from build123d import *

# Parameters (mm, degrees)
PAD006_DEPTH         = 1
SKETCH010_W          = 9.75
SKETCH010_H          = 7
PAD007_DEPTH         = 1.85
SKETCH012_R          = 1.875
PAD005_DEPTH         = 2
POCKET_DEPTH         = 9.001
POCKET001_DEPTH      = 4.876
POCKET001_DEPTH_BACK = -4.876
CHAMFER_SIZE         = 0.3


with BuildPart() as part:
    # Sketch013 → Pad006 (new body)
    with BuildSketch(Plane.XZ):
        with BuildLine():
            ThreePointArc((1.274755, -5.005), (0, -4.505), (-1.274755, -5.005))
            Line((-1.274755, -5.005), (-3.875, -5.005))
            ThreePointArc((-3.875, -5.005), (-4.582107, -5.297893), (-4.875, -6.005))
            Line((-4.875, -6.005), (-4.875, -7.255))
            ThreePointArc((-4.875, -7.255), (-4.582107, -7.962107), (-3.875, -8.255))
            Line((-3.875, -8.255), (3.875, -8.255))
            ThreePointArc((3.875, -8.255), (4.582107, -7.962107), (4.875, -7.255))
            Line((4.875, -7.255), (4.875, -6.005))
            ThreePointArc((4.875, -6.005), (4.582107, -5.297893), (3.875, -5.005))
            Line((3.875, -5.005), (1.274755, -5.005))
        make_face()
    extrude(amount=PAD006_DEPTH)

    # Sketch010 → Pad007 (join)
    with BuildSketch(Plane.XZ):
        with Locations((0, -5.5)):
            Rectangle(SKETCH010_W, SKETCH010_H)
    extrude(amount=-PAD007_DEPTH)

    # Sketch012 → Pad005 (join)
    with BuildSketch(Plane.XZ.offset(1)):
        with Locations((0, -6.38)):
            Circle(SKETCH012_R)
    extrude(amount=PAD005_DEPTH)

    # Sketch → Pocket (cut, through all)
    with BuildSketch(Plane.XY):
        Polygon((-1.275, 3.6), (-1.275, 1.6), (1.275, 1.6), (1.275, 3.6), (4.875, 0), (4.875, 5), (-4.875, 5), (-4.875, 0), align=None)
    extrude(amount=-POCKET_DEPTH, mode=Mode.SUBTRACT)

    # Sketch014 → Pocket001 (cut, two sides)
    with BuildSketch(Plane.YZ) as pocket001_sk:
        Polygon((0, 0), (0, -2), (4, -6), (4, 0), align=None)
    extrude(amount=-POCKET001_DEPTH, mode=Mode.SUBTRACT)
    extrude(pocket001_sk.sketch, amount=-POCKET001_DEPTH_BACK, mode=Mode.SUBTRACT)

    # Chamfer
    chamfer_edges = [part.edges().sort_by_distance(p)[0] for p in [
        (-1.875, -3, -6.38),
        (0, 1.6, -3.6),
        (-4.875, 0, -4.0025),
        (-4.875, 0, -8.1275),
        (4.875, 0, -4.0025),
        (4.875, 0, -8.1275),
        (0, 0, -9),
        (0, 0, -2),
    ]]
    chamfer(chamfer_edges, length=CHAMFER_SIZE)


solid = part.part
The listing builds one solid part. Answer for the finished solid, in the listing's coordinates (mm). A direction names the side the tool comes from. Give positions to 0.01 mm unless a question says otherwise; leave off trailing zeros. Write each loop counter-clockwise with the first axis right and the second up, starting at its lowest first coordinate (ties: lowest second). Pieces come first, ordered by that corner, then holes.
1) Find the intervals of material crossed by L1, parallel to Y at x = 0, z = -6.5; L2, parallel to Y at x = 1.75, z = -4.25; L3, parallel to Z at x = 2.25, y = -0.05 (3 decimals), in increasing order.
2) Section A-A (z = -6.38) is taken. Write down the section's boundary in (x, y) (3 decimals), and give its area (3 significant figures).
3) A tool of negligible diameter and unlimited length cuts with its end or side. For faces 4 (the face through (4.59, -0.52, -5.306)), 5 (the face through (-0.1, -0.5, -8.255)), 6 (the face through (-2.6, -0.5, -5.005)), from which of +Z, -Z, +X, -X, +Y, -Y can it reach the whole face along a straight path? Write none if from no direction.
4) Section B-B (y = -0.4) is taken. Write down the section's boundary in (x, z) (3 decimals).
5) Section D-D (y = -1.55) is taken. Write down the section's boundary in (x, z) (3 decimals), and give its area (3 significant figures).
6) Given P1, Ø1.1, axis at x = -2.5, y = -0.5, coming from the +Z side; P2, Ø1, axis at x = -0.5, z = -7.5, coming from the +Y side; P3, Ø1.5, axis at y = 0.5, z = -5, coming from the +X side, each flat-ended and moving along its own axis, determine where each tip first touches the part or whether it passes through.
7) Section C-C (x = -2.75) is taken. Write down the section's boundary in (y, z) (3 decimals).
8) For a pull along X with two mould halves and no side action, classify faces 1 (the face through (-2, 1.85, -6)), 2 (the face through (-3.963, 0.912, -6.313)), 3 (the face through (0, 1.6, -6)) as pulls with the +X half, pulls with the -X half, needs draft (parallel to the pull), parting line crosses it, or undercut.
Response:
1. L1: y = -3 to 1.6
1. L2: y = 0 to 1.85
1. L3: z = -8.255 to -5.005
2. outline: (-4.875, -1) - (-1.875, -1) - (-1.875, -2.7) - (-1.575, -3) - (1.575, -3) - (1.875, -2.7) - (1.875, -1) - (4.875, -1) - (4.875, 0) - (3.025, 1.85) - (1.275, 1.85) - (1.275, 1.6) - (-1.275, 1.6) - (-1.275, 1.85) - (-3.025, 1.85) - (-4.875, 0) - close
2. area: 31.1 mm2
3. face 4: +Z, +X, -Y
3. face 5: -Z, +X, -X, -Y
3. face 6: +Z, -X, -Y
4. outline: (-4.875, -7.255) arc R1 ccw to (-3.875, -8.255) - (3.875, -8.255) arc R1 ccw to (4.875, -7.255) - (4.875, -6.005) arc R1 ccw to (3.875, -5.005) - (1.275, -5.005) arc R1.875 ccw to (-1.275, -5.005) - (-3.875, -5.005) arc R1 ccw to (-4.875, -6.005) - close
5. outline: circle Ø3.75 at (0, -6.38)
5. area: 11.0 mm2
6. P1: stops at z = -2.28
6. P2: stops at y = 1.6
6. P3: stops at x = 4.8
7. outline: (-1, -8.255) - (0, -8.255) - (0, -8.7) - (0.3, -9) - (1.85, -9) - (1.85, -3.85) - (0.212, -2.212) - (0, -2.3) - (0, -5.005) - (-1, -5.005) - close
8. face 1: needs draft
8. face 2: pulls with the -X half
8. face 3: undercut
